from build123d import *

# Parameters (mm, degrees)
SKETCH1_W          = 266
SKETCH1_H          = 25.5
BASE_FLANGE1_DEPTH = 1
HEM1_START         = -133
HEM1_DEPTH         = 266
HEM1_2_DEPTH       = 266
CUT_EXTRUDE1_START = -134.703262862
SKETCH8_W          = 14
SKETCH8_H          = 6
CUT_EXTRUDE1_DEPTH = 259.406525724
LPATTERN1_COUNT    = 11
LPATTERN1_PITCH    = 28
CHAMFER1_SIZE      = 0.5
SKETCH10_W         = 266
SKETCH10_H         = 4
CUT_EXTRUDE3_DEPTH = 10
SKETCH9_R          = 2
CUT_EXTRUDE2_DEPTH = 10
LPATTERN2_COUNT    = 5
LPATTERN2_PITCH    = 60
CHAMFER2_SIZE      = 1


# Read off the part's stored shape, not the designer's step: Hem1
# Sheet-metal steps are written as plain solids
with BuildPart() as part:
    # Sketch1 → Base-Flange1 (new body)
    with BuildSketch(Plane(origin=(0, 0, 0), x_dir=(1, 0, 0), z_dir=(0, 1, 0))):
        Rectangle(SKETCH1_W, SKETCH1_H)
    extrude(amount=-BASE_FLANGE1_DEPTH)

    # Hem1 outline → Hem1 (cut)
    with BuildSketch(Plane.YZ.offset(HEM1_START)):
        with BuildLine():
            Line((0, -12.75), (0, -11.986067977))
            ThreePointArc((0, -11.986067977), (-0.738612788, -10.974744871), (-1, -9.75))
            Line((-1, -9.75), (-1, -12.75))
            Line((-1, -12.75), (0, -12.75))
        make_face()
    extrude(amount=HEM1_DEPTH, mode=Mode.SUBTRACT)

    # Hem1 2 outline → Hem1 2 (add)
    with BuildSketch(Plane.YZ.offset(HEM1_START)):
        with BuildLine():
            Line((0.732145215, -7.031076639), (1.154763477, -7.937384426))
            ThreePointArc((1.154763477, -7.937384426), (3.686782892, -10.824599218), (0, -9.75))
            Line((0, -9.75), (0, -11.986067977))
            ThreePointArc((0, -11.986067977), (4.967777538, -10.18851623), (0.732145215, -7.031076639))
        make_face()
    extrude(amount=HEM1_2_DEPTH)

    # Sketch8 → Cut-Extrude1 (cut)
    with BuildSketch(Plane(origin=(0, 0, 0), x_dir=(1, 0, 0), z_dir=(0, 1, 0)).offset(CUT_EXTRUDE1_START)):
        with Locations((126, 9.75)):
            Rectangle(SKETCH8_W, SKETCH8_H)
    cut_extrude1 = extrude(amount=CUT_EXTRUDE1_DEPTH, mode=Mode.SUBTRACT)

    # LPattern1: Cut-Extrude1 ×11
    with Locations(*[(-i * LPATTERN1_PITCH, 0, 0) for i in range(1, LPATTERN1_COUNT)]):
        add(cut_extrude1, mode=Mode.SUBTRACT)

    # Chamfer1
    chamfer1_edges = [part.edges().sort_by_distance(p)[0] for p in [
        (-133, 0, 3),
        (0, 0, 12.75),
        (133, 0, 3),
    ]]
    chamfer(chamfer1_edges, length=CHAMFER1_SIZE)

    # Sketch10 → Cut-Extrude3 (cut)
    with BuildSketch(Plane(origin=(0, 0, 0), x_dir=(1, 0, 0), z_dir=(0, 1, 0))):
        with Locations((0, -10.75)):
            Rectangle(SKETCH10_W, SKETCH10_H)
    extrude(amount=-CUT_EXTRUDE3_DEPTH, mode=Mode.SUBTRACT)

    # Sketch9 → Cut-Extrude2 (cut)
    with BuildSketch(Plane(origin=(0, 0, 0), x_dir=(1, 0, 0), z_dir=(0, 1, 0))):
        with Locations(Location((-120, -1.25, 0), (0, 0, 270))):
            Circle(SKETCH9_R)
    cut_extrude2 = extrude(amount=-CUT_EXTRUDE2_DEPTH, mode=Mode.SUBTRACT)

    # LPattern2: Cut-Extrude2 ×5
    with Locations(*[(i * LPATTERN2_PITCH, 0, 0) for i in range(1, LPATTERN2_COUNT)]):
        add(cut_extrude2, mode=Mode.SUBTRACT)

    # Chamfer2
    chamfer2_edges = [part.edges().sort_by_distance(p)[0] for p in [
        (-120, 0, -0.75),
        (-60, 0, -0.75),
        (0, 0, -0.75),
        (60, 0, -0.75),
        (120, 0, -0.75),
    ]]
    chamfer(chamfer2_edges, length=CHAMFER2_SIZE - 0.0001)  # a hair under: the kernel refuses the full size


solid = part.part
Check sheet for the modelled part. Datum: model origin and axes. Units: mm. A direction names the side the tool comes from. Give positions to 0.01 mm unless a question says otherwise; leave off trailing zeros. Loops run counter-clockwise (first coordinate to the right, second up) from the corner with the lowest first, then second, coordinate; pieces in that order, holes last. Notation, with made-up numbers: M 17,69 L 59,69 A33 ccw 59,104 Z; hole C 0.5,-6 d8. An arc over 180 degrees is marked long. Return JSON: item names as keys, results as strings. Group by question number.
1. Thickness scan on L1, parallel to X at y = -0.95, z = 1.25; L2, parallel to Z at x = 117, y = 2.4; L3, parallel to Y at x = 108, z = 3. Record the ranges inside material, lowest first.
2. Cross-section at B-B on y = 3.1. State how many separate pieces and enclosed holes the cut face has, plus the area to 3 significant figures.
3. Cross-section at C-C on x = 11.5. Record the boundary of the cut face in (y, z), plus the area to 3 significant figures.
4. Go/stop test with flat-tipped pins: pin 1 (0.5 mm diameter, centred on x = -68.5, y = -0.5, fed in from -Z); pin 2 (5 mm diameter, centred on x = 0, z = 1.25, fed in from +Y); pin 3 (6.5 mm diameter, centred on x = 60, z = 1.25, fed in from +Y). Record where each tip stops, or that it passes through.
5. Tool access check on faces 1 (the flat face through (-2, -1, -1)), 2 (the flat face through (119, 1.3, -7.7)), 3 (the flat face through (35, 1.3, -7.7)). Record the directions out of +Z, -Z, +X, -X, +Y, -Y that give a thin tool (end or side, any length) a straight path to the whole face; none if there is none.
6. Cross-section at A-A on x = 108. Record the boundary of the cut face in (y, z).
Return value:
{
 "1": {"L1": "-133 to -122.05, -117.95 to -62.05, -57.95 to -2.05, 2.05 to 57.95, 62.05 to 117.95, 122.05 to 133", "L2": "-12.72 to -11.71, -7.79 to -6.78", "L3": "-1 to 0"},
 "2": {"separate pieces": "18", "enclosed holes": "0", "area": "282 mm^2"},
 "3": {"outline": "M -1,-6.75 L 0,-6.75 L 0,8.75 L -1,8.75 Z", "area": "15.5 mm^2"},
 "4": {"pin 1": "z = -6.75", "pin 2": "y = -0.5", "pin 3": "y = 0"},
 "5": {"face 1": "+Z, -Z, +X, -X, -Y", "face 2": "-Z, +X, +Y, -Y", "face 3": "-Z, +Y, -Y"},
 "6": {"outline": "M -1,-9.75 A3 ccw long 0.73,-7.03 L 1.15,-7.94 A2 cw long 0,-9.75 L 0,8.75 L -1,8.75 Z"}
}
